Here's how the part is built. I have some questions about the finished solid (model axes, mm). A direction names the side the tool comes from. Give positions to 0.01 mm unless a question says otherwise; leave off trailing zeros. Order: outer loops, then holes, each group sorted by start corner. A loop starts at its lowest first (then second) coordinate and runs counter-clockwise, first axis right, second up. Notation, with made-up numbers: (44, -18) - (80, -18) arc R15 cw to (80, -7) - close; hole circle Ø9 at (-10.75, 82.5). An arc over 180 degrees is marked (long way). One line per question, with ' | ' between items.
from build123d import *

# Parameters (mm, degrees)
SKETCH_1_W          = 60
SKETCH_1_H          = 50
EXTRUDE_1_DEPTH     = 9.5
FILLET_1_R          = 3
SKETCH_2_R          = 4
CUT_EXTRUDE_1_DEPTH = 1
SKETCH_5_R          = 1.9
CUT_EXTRUDE_3_DEPTH = 41.190172928
SKETCH_6_R          = 1.4
CUT_EXTRUDE_4_DEPTH = 41.190172928
CUT_EXTRUDE_START   = -4
SKETCH_7_R          = 4
SKETCH_7_R_2        = 3
CUT_EXTRUDE_5_DEPTH = 4


with BuildPart() as part:
    # 草图1 → 凸台-拉伸1 (new body)
    with BuildSketch(Plane(origin=(0, 0, 0), x_dir=(1, 0, 0), z_dir=(0, 1, 0))):
        Rectangle(SKETCH_1_W, SKETCH_1_H)
    extrude(amount=EXTRUDE_1_DEPTH)

    # 圆角1
    fillet_1_edges = [part.edges().sort_by_distance(p)[0] for p in [
        (30, 4.75, 25),
        (-30, 4.75, 25),
    ]]
    fillet(fillet_1_edges, radius=FILLET_1_R)

    # 草图2 → 切除-拉伸1 (cut)
    with BuildSketch(Plane(origin=(0, 9.5, 0), x_dir=(1, 0, 0), z_dir=(0, 1, 0))):
        with Locations(Location((-20, -15, 0), (0, 0, 270))):
            Circle(SKETCH_2_R)
        with Locations(Location((20, -15, 0), (0, 0, 270))):
            Circle(SKETCH_2_R)
    extrude(amount=-CUT_EXTRUDE_1_DEPTH, mode=Mode.SUBTRACT)

    # 草图5 → 切除-拉伸3 (cut, through all)
    with BuildSketch(Plane(origin=(0, 9.5, 0), x_dir=(1, 0, 0), z_dir=(0, 1, 0))):
        with Locations(Location((-20, -15, 0), (0, 0, 270))):
            Circle(SKETCH_5_R)
        with Locations(Location((20, -15, 0), (0, 0, 270))):
            Circle(SKETCH_5_R)
    extrude(amount=-CUT_EXTRUDE_3_DEPTH, mode=Mode.SUBTRACT)

    # 草图6 → 切除-拉伸4 (cut, through all)
    with BuildSketch(Plane.XZ):
        with Locations(Location((-25, -21, 0), (0, 0, 270))):
            Circle(SKETCH_6_R)
        with Locations(Location((-25, -2, 0), (0, 0, 270))):
            Circle(SKETCH_6_R)
        with Locations(Location((25.25, -21, 0), (0, 0, 270))):
            Circle(SKETCH_6_R)
        with Locations(Location((25.25, -2, 0), (0, 0, 270))):
            Circle(SKETCH_6_R)
    extrude(amount=-CUT_EXTRUDE_4_DEPTH, mode=Mode.SUBTRACT)

    # 草图7 → 切除-拉伸5 (cut)
    with BuildSketch(Plane.XZ.offset(CUT_EXTRUDE_START)):
        with Locations(Location((-20, 15, 0), (0, 0, 90))):
            Circle(SKETCH_7_R)
        with Locations(Location((20, 15, 0), (0, 0, 90))):
            Circle(SKETCH_7_R)
        with Locations(Location((25.25, -2, 0), (0, 0, 270))):
            Circle(SKETCH_7_R_2)
        with Locations(Location((25.25, -21, 0), (0, 0, 270))):
            Circle(SKETCH_7_R_2)
        with Locations(Location((-25, -21, 0), (0, 0, 270))):
            Circle(SKETCH_7_R_2)
        with Locations(Location((-25, -2, 0), (0, 0, 270))):
            Circle(SKETCH_7_R_2)
    extrude(amount=CUT_EXTRUDE_5_DEPTH, mode=Mode.SUBTRACT)


solid = part.part
1) I'm going to push flat-ended pins straight in: P1, Ø3, axis at x = 25.25, z = -2, coming from the -Y side; P2, Ø2.5, axis at x = -19.5, z = 17, coming from the +Y side. Where does each tip first touch, or does it pass through?
Model answer:
P1: stops at y = 4 | P2: stops at y = 8.5
2) I want a section at A-A (z = -21). List the corners of the cut face in (x, y) for me.
Model answer:
outline: (-30, 0) - (-28, 0) - (-28, 4) - (-26.4, 4) - (-26.4, 9.5) - (-30, 9.5) - close; (-23.6, 4) - (-22, 4) - (-22, 0) - (22.25, 0) - (22.25, 4) - (23.85, 4) - (23.85, 9.5) - (-23.6, 9.5) - close; (26.65, 4) - (28.25, 4) - (28.25, 0) - (30, 0) - (30, 9.5) - (26.65, 9.5) - close
3) I want a section at C-C (y = 6.5). List the corners of the cut face in (x, z) for me, plus the area to 3 significant figures.
Model answer:
outline: (-30, -25) - (30, -25) - (30, 22) arc R3 ccw to (27, 25) - (-27, 25) arc R3 ccw to (-30, 22) - close; hole circle Ø2.8 at (-25, -21); hole circle Ø2.8 at (-25, -2); hole circle Ø3.8 at (-20, 15); hole circle Ø3.8 at (20, 15); hole circle Ø2.8 at (25.25, -21); hole circle Ø2.8 at (25.25, -2) | area: 2,950 mm2
4) I want a section at B-B (x = 20). List the corners of the cut face in (y, z) for me, plus the area to 3 significant figures.
Model answer:
outline: (0, -25) - (9.5, -25) - (9.5, 11) - (8.5, 11) - (8.5, 13.1) - (4, 13.1) - (4, 11) - (0, 11) - close; (0, 19) - (4, 19) - (4, 16.9) - (8.5, 16.9) - (8.5, 19) - (9.5, 19) - (9.5, 25) - (0, 25) - close | area: 418 mm2
5) Please list where these lines run through material, in increasing order: L1, parallel to X at y = 7.3, z = -2; L2, parallel to X at y = 2.8, z = -21; L3, parallel to Z at x = 25.5, y = 5.75.
Model answer:
L1: x = -30 to -26.4, -23.6 to 23.85, 26.65 to 30 | L2: x = -30 to -28, -22 to 22.25, 28.25 to 30 | L3: z = -25 to -22.38, -19.62 to -3.38, -0.62 to 25
6) Thinking about a two-plate mould opening in X: for faces 4 (the face through (-30, 5, -1)), 5 (the face through (0, 0, 0)), 6 (the face through (-25, 2, -18)), which applies, +X half, -X half, draft (parallel to the pull), parting line (faces both ways), or undercut?
Model answer:
face 4: -X half | face 5: draft | face 6: undercut
7) On a 3-axis mill with a long thin cutter (end or side, diameter ignored), from which of +Z, -Z, +X, -X, +Y, -Y can I reach the whole of each face in a straight line? I mean faces 1 (the face through (0, 5, 25)), 2 (the face through (24, 4, -22)), 3 (the face through (-22, 8.5, 16)). Say none if no direction works.
Model answer:
face 1: +Z, +X, -X, +Y, -Y | face 2: -Y | face 3: +Y
